from build123d import *

# Parameters (mm, degrees)
CROQUIS1_W              = 34
CROQUIS1_H              = 10
SALIENTE_EXTRUIR1_DEPTH = 3.6
CROQUIS2_W              = 34
CROQUIS2_H              = 10
SALIENTE_EXTRUIR2_DEPTH = 1
CROQUIS3_W              = 6.6
CROQUIS3_H              = 6.6
CROQUIS3_W_2            = 3.6
CROQUIS3_H_2            = 3.6
SALIENTE_EXTRUIR3_DEPTH = 4


with BuildPart() as part:
    # Croquis1 → Saliente-Extruir1 (new body)
    with BuildSketch(Plane.XY):
        with Locations((-28.217187331, 0.443569554)):
            Rectangle(CROQUIS1_W, CROQUIS1_H)
        with BuildLine():
            Line((-25.840984713, 3.661280093), (-14.217187331, 2.443569554))
            ThreePointArc((-14.217187331, 2.443569554), (-12.217187331, 0.443569554), (-14.217187331, -1.556430446))
            Line((-14.217187331, -1.556430446), (-25.840984713, -2.774140986))
            ThreePointArc((-25.840984713, -2.774140986), (-28.217187331, -3.556430446), (-30.593389949, -2.774140986))
            Line((-30.593389949, -2.774140986), (-42.217187331, -1.556430446))
            ThreePointArc((-42.217187331, -1.556430446), (-44.217187331, 0.443569554), (-42.217187331, 2.443569554))
            Line((-42.217187331, 2.443569554), (-30.593389949, 3.661280093))
            ThreePointArc((-30.593389949, 3.661280093), (-28.217187331, 4.443569554), (-25.840984713, 3.661280093))
        make_face(mode=Mode.SUBTRACT)
    extrude(amount=SALIENTE_EXTRUIR1_DEPTH)

    # Croquis2 → Saliente-Extruir2 (add)
    with BuildSketch(Plane.XY.offset(3.6)):
        with Locations((-28.217187331, 0.443569554)):
            Rectangle(CROQUIS2_W, CROQUIS2_H)
    extrude(amount=SALIENTE_EXTRUIR2_DEPTH)

    # Croquis3 → Saliente-Extruir3 (add)
    with BuildSketch(Plane.XY.offset(4.6)):
        with Locations((-28.217187331, 0.443569554)):
            Rectangle(CROQUIS3_W, CROQUIS3_H)
        with Locations((-28.217187331, 0.443569554)):
            Rectangle(CROQUIS3_W_2, CROQUIS3_H_2, mode=Mode.SUBTRACT)
    extrude(amount=SALIENTE_EXTRUIR3_DEPTH)


solid = part.part
Work out the finished part from the listing and answer in its coordinate system (mm). A direction names the side the tool comes from. Give positions to 0.01 mm unless a question says otherwise; leave off trailing zeros. Loops run counter-clockwise (first coordinate to the right, second up) from the corner with the lowest first, then second, coordinate; pieces in that order, holes last. Notation, with made-up numbers: (0, 69.25) - (22, 69.25) arc R18 ccw to (22, 80.25) - close; hole circle Ø6 at (22, 72). An arc over 180 degrees is marked (long way). Answer in a Markdown table with one row per item. Add a question column.
Q1. Consider line 1 along X through (y, z) = (0.5, 1.75); line 2 along Z through (x, y) = (-42.5, -2.75); line 3 along Z through (x, y) = (-43, 2). Determine where each line is inside the solid, lowest interval first.
Q2. Each of these flat-tipped pins is pushed along its axis until it touches: P1, Ø4, axis at x = -24, y = -0.5, coming from the -Z side; P2, Ø1.2, axis at x = -29, z = 6, coming from the -Y side; P3, Ø1.5, axis at x = -17.5, y = -3, coming from the +Z side; P4, Ø4, axis at x = -41, z = 7, coming from the +Y side (3 decimals). Where does it stop, or does it pass through?
Q3. The part is cut by section B-B (y = 0.5). Determine the outline of the cut face in (x, z).
Q4. Determine the mould class of faces 6 (the flat face through (-19.948, -2.157, 1.775)), 7 (the flat face through (-11.217, 0, 2)), 8 (the flat face through (-28, -4.556, 2)) for opening direction X: released by +X, released by -X, zero draft, split by the parting line, or undercut.
Q5. The part is cut by section C-C (x = -33). Determine the outline of the cut face in (y, z), and give its area (3 significant figures).
Q6. The part is cut by section D-D (z = 5.5). Determine the outline of the cut face in (x, y).
Q7. The part is cut by section A-A (z = 1.5). Determine the outline of the cut face in (x, y), and give its area (3 significant figures).
Q8. A tool of negligible diameter and unlimited length cuts with its end or side. For faces 1 (the flat face through (-28, 0, 4.6)), 2 (the flat face through (-31.517, 0, 7)), 3 (the flat face through (-24.917, 0, 7)), 4 (the flat face through (-28, 5, 0)), 5 (the cylindrical face through (-28.182, -3.556, 1.775)), from which of +Z, -Z, +X, -X, +Y, -Y can it reach the whole face along a straight path? Write none if from no direction.
Solution:
| question | item | result |
|---|---|---|
| 1 | line 1 | x = -45.22 to -44.22, -12.22 to -11.22 |
| 1 | line 2 | z = 0 to 4.6 |
| 1 | line 3 | z = 3.6 to 4.6 |
| 2 | P1 | stops at z = 3.6 |
| 2 | P2 | stops at y = -2.86 |
| 2 | P3 | stops at z = 4.6 |
| 2 | P4 | passes through |
| 3 | outline | (-45.22, 0) - (-44.22, 0) - (-44.22, 3.6) - (-12.22, 3.6) - (-12.22, 0) - (-11.22, 0) - (-11.22, 4.6) - (-24.92, 4.6) - (-24.92, 8.6) - (-26.42, 8.6) - (-26.42, 4.6) - (-30.02, 4.6) - (-30.02, 8.6) - (-31.52, 8.6) - (-31.52, 4.6) - (-45.22, 4.6) - close |
| 4 | face 6 | undercut |
| 4 | face 7 | released by +X |
| 4 | face 8 | zero draft |
| 5 | outline | (-4.56, 0) - (-2.52, 0) - (-2.52, 3.6) - (3.41, 3.6) - (3.41, 0) - (5.44, 0) - (5.44, 4.6) - (-4.56, 4.6) - close |
| 5 | area | 24.6 mm² |
| 6 | outline | (-31.52, -2.86) - (-24.92, -2.86) - (-24.92, 3.74) - (-31.52, 3.74) - close; hole (-30.02, -1.36) - (-26.42, -1.36) - (-26.42, 2.24) - (-30.02, 2.24) - close |
| 7 | outline | (-45.22, -4.56) - (-11.22, -4.56) - (-11.22, 5.44) - (-45.22, 5.44) - close; hole (-42.22, -1.56) - (-30.59, -2.77) arc R4 ccw to (-25.84, -2.77) - (-14.22, -1.56) arc R2 ccw to (-14.22, 2.44) - (-25.84, 3.66) arc R4 ccw to (-30.59, 3.66) - (-42.22, 2.44) arc R2 ccw to start |
| 7 | area | 170 mm² |
| 8 | face 1 | +Z |
| 8 | face 2 | +Z, -X, +Y, -Y |
| 8 | face 3 | +Z, +X, +Y, -Y |
| 8 | face 4 | -Z, +X, -X, +Y, -Y |
| 8 | face 5 | -Z |
